```python
from build123d import *

# Parameters (mm, degrees)
F0_R     = 1.65
F0_R_2   = 1.5
F0_R_3   = 3.55
F1_DEPTH = 4
F2_SIZE2 = 1.5
F2_SIZE  = 1.5


with BuildPart() as f1:
    # F0 (on Top) → F1 (new body)
    with BuildSketch(Plane.XY):
        with BuildLine():
            ThreePointArc((12, 8), (10.828427, 10.828427), (8, 12))
            Line((8, 12), (-8, 12))
            ThreePointArc((-8, 12), (-10.828427, 10.828427), (-12, 8))
            Line((-12, 8), (-12, -8))
            ThreePointArc((-12, -8), (-10.828427, -10.828427), (-8, -12))
            Line((-8, -12), (8, -12))
            ThreePointArc((8, -12), (10.828427, -10.828427), (12, -8))
            Line((12, -8), (12, 8))
        make_face()
        with Locations((-8, -8)):
            Circle(F0_R, mode=Mode.SUBTRACT)
        with Locations((0, -8.5)):
            Circle(F0_R_2, mode=Mode.SUBTRACT)
        with Locations((8, -8)):
            Circle(F0_R, mode=Mode.SUBTRACT)
        with Locations((-8, 8)):
            Circle(F0_R, mode=Mode.SUBTRACT)
        Circle(F0_R_3, mode=Mode.SUBTRACT)
        with Locations((0, 8.5)):
            Circle(F0_R_2, mode=Mode.SUBTRACT)
        with Locations((8, 8)):
            Circle(F0_R, mode=Mode.SUBTRACT)
    extrude(amount=F1_DEPTH)

    # F2
    f2_edges = [f1.edges().sort_by_distance(p)[0] for p in [
        (-1.5, 8.5, 4),
        (-1.5, -8.5, 4),
    ]]
    chamfer(f2_edges, length=F2_SIZE, length2=F2_SIZE2)


solid = f1.part
```
The listing builds one solid part. Answer for the finished solid, in the listing's coordinates (mm). Give positions to 0.01 mm unless a question says otherwise; leave off trailing zeros. Loops run counter-clockwise (first coordinate to the right, second up) from the corner with the lowest first, then second, coordinate; pieces in that order, holes last. Notation, with made-up numbers: (53.25, 69.5) - (89.25, 69.5) arc R16 ccw to (89.25, 93.5) - close; hole circle Ø4 at (-36.75, -19.75). An arc over 180 degrees is marked (long way). Return JSON: item names as keys, results as strings. Group by question number.
1. Find section A-A (y = 0). Write down the section's boundary in (x, z).
2. Given pin 1 Ø3 at (x, y) = (8, -8) entering from +Z; pin 2 Ø4 at (x, y) = (0, -8.5) entering from +Z, each flat-ended and moving along its own axis, determine where each tip first touches the part or whether it passes through.
3. Straight lines are drawn through the part: line 1 (Y direction, x = 0, z = 0.6); line 2 (X direction, y = 7.5, z = 2.3); line 3 (X direction, y = -6.5, z = 3.45). For each, find the intervals that lie inside material, in ascending order. Write a range as [from, to].
4. Find section C-C (z = 1.5). Write down the section's boundary in (x, y), then the cut area to 3 significant figures.
5. Find section B-B (x = 0). Write down the section's boundary in (y, z).
6. Determine the mould class of faces 1 (the cylindrical face through (6.69, -9, 1.97)), 2 (the cylindrical face through (-10.859, -10.797, 1.972)), 3 (the flat face through (12, 0, 2)) for opening direction X: pulls with the +X half, pulls with the -X half, needs draft (parallel to the pull), parting line crosses it, or undercut.
7. Find section D-D (y = -8.5). Write down the section's boundary in (x, z), then the cut area to 3 significant figures.
Verdict:
{
 "1": {"outline": "(-12, 0) - (-3.55, 0) - (-3.55, 4) - (-12, 4) - close; (3.55, 0) - (12, 0) - (12, 4) - (3.55, 4) - close"},
 "2": {"pin 1": "passes through", "pin 2": "stops at z = 3"},
 "3": {"line 1": "y = [-12, -10], [-7, -3.55], [3.55, 7], [10, 12]", "line 2": "x = [-12, -9.57], [-6.43, -1.12], [1.12, 6.43], [9.57, 12]", "line 3": "x = [-12, -8.69], [-7.31, -1.42], [1.42, 7.31], [8.69, 12]"},
 "4": {"outline": "(-12, -8) arc R4 ccw to (-8, -12) - (8, -12) arc R4 ccw to (12, -8) - (12, 8) arc R4 ccw to (8, 12) - (-8, 12) arc R4 ccw to (-12, 8) - close; hole circle Ø3.3 at (-8, -8); hole circle Ø3.3 at (-8, 8); hole circle Ø7.1 at (0, 0); hole circle Ø3 at (0, -8.5); hole circle Ø3 at (0, 8.5); hole circle Ø3.3 at (8, -8); hole circle Ø3.3 at (8, 8)", "area": "474 mm^2"},
 "5": {"outline": "(-12, 0) - (-10, 0) - (-10, 2.5) - (-11.5, 4) - (-12, 4) - close; (-7, 0) - (-3.55, 0) - (-3.55, 4) - (-5.5, 4) - (-7, 2.5) - close; (3.55, 0) - (7, 0) - (7, 2.5) - (5.5, 4) - (3.55, 4) - close; (10, 0) - (12, 0) - (12, 4) - (11.5, 4) - (10, 2.5) - close"},
 "6": {"face 1": "undercut", "face 2": "pulls with the -X half", "face 3": "pulls with the +X half"},
 "7": {"outline": "(-11.97, 0) - (-9.57, 0) - (-9.57, 4) - (-11.97, 4) - close; (-6.43, 0) - (-1.5, 0) - (-1.5, 2.5) - (-3, 4) - (-6.43, 4) - close; (1.5, 0) - (6.43, 0) - (6.43, 4) - (3, 4) - (1.5, 2.5) - close; (9.57, 0) - (11.97, 0) - (11.97, 4) - (9.57, 4) - close", "area": "56.3 mm^2"}
}
